```python
from build123d import *

# Parameters (mm, degrees)
EXTRUIR_L_MINA1_DEPTH           = 25
REDONDEO1_R                     = 5
CROQUIS2_R                      = 3
CORTAR_EXTRUIR1_DEPTH           = 41.555257948
REDONDEO2_RADIUS                = 3
REDONDEO2_LENGTH                = 50
REDONDEO3_R                     = 2
REDONDEO1_OF_SIMETR_A1_R        = 5
REDONDEO2_OF_SIMETR_A1_2_RADIUS = 3
REDONDEO2_OF_SIMETR_A1_2_LENGTH = 50
REDONDEO3_OF_SIMETR_A1_R        = 2
TALADRO2_D                      = 5.6
REDONDEO4_R                     = 1


with BuildPart() as part:
    # Croquis1 → Extruir-Lámina1 (new, symmetric)
    with BuildSketch(Plane.XY):
        Polygon((0, 0), (8.029231721, 0), (20, -6.300526927), (31.305467696, -0.350165014), (28.510946527, 4.959321914), (20, 0.479789229), (9.511803576, 6), (0, 6), align=None)
    extruir_l_mina1 = extrude(amount=EXTRUIR_L_MINA1_DEPTH, both=True)

    # Redondeo1
    redondeo1_edges = [part.edges().sort_by_distance(p)[0] for p in [
        (20, 0.479789229, 0),
    ]]
    fillet(redondeo1_edges, radius=REDONDEO1_R)

    # Croquis2 → Cortar-Extruir1 (cut, symmetric)
    with BuildSketch(Plane.XY):
        with Locations((20, -6.300526927)):
            Circle(CROQUIS2_R)
    cortar_extruir1 = extrude(amount=CORTAR_EXTRUIR1_DEPTH, both=True, mode=Mode.SUBTRACT)

    # Redondeo2: full round fillet: the end face becomes a half cylinder, R = half its width
    redondeo2_face = Plane((29.908207112, 2.30457845, 0), x_dir=(0, 0, 1), z_dir=(0.884914487987, 0.465753528113, 0))  # on the end face: x along it, z out of the body
    redondeo2_slab = redondeo2_face.offset(-REDONDEO2_RADIUS / 2) * Box(REDONDEO2_LENGTH, 2 * REDONDEO2_RADIUS, REDONDEO2_RADIUS, mode=Mode.PRIVATE)  # the body's end, R deep
    redondeo2_round = Plane((27.253463648, 0.907317866, 0), x_dir=(0.884914487987, 0.465753528113, 0), z_dir=(0, 0, 1)) * Cylinder(REDONDEO2_RADIUS, REDONDEO2_LENGTH, mode=Mode.PRIVATE)  # its axis R under the face
    add(redondeo2_slab - redondeo2_round, mode=Mode.SUBTRACT)

    # Redondeo3
    redondeo3_edges = [part.edges().sort_by_distance(p)[0] for p in [
        (22.654743464, -4.903266343, 0),
        (17.345256536, -4.903266343, 0),
    ]]
    fillet(redondeo3_edges, radius=REDONDEO3_R)

    # Simetría1: Extruir-Lámina1, Cortar-Extruir1 across plane
    add(extruir_l_mina1.mirror(Plane(origin=(0, 0, 0), x_dir=(0, 0, 1), z_dir=(1, 0, 0))))
    add(cortar_extruir1.mirror(Plane(origin=(0, 0, 0), x_dir=(0, 0, 1), z_dir=(1, 0, 0))), mode=Mode.SUBTRACT)

    # Redondeo1 of Simetría1
    redondeo1_of_simetr_a1_edges = [part.edges().sort_by_distance(p)[0] for p in [
        (-20, 0.479789229, 0),
    ]]
    fillet(redondeo1_of_simetr_a1_edges, radius=REDONDEO1_OF_SIMETR_A1_R)

    # Redondeo2 of Simetr_a1 2: full round fillet: the end face becomes a half cylinder, R = half its width
    redondeo2_of_simetr_a1_2_face = Plane((-29.908207112, 2.30457845, 0), x_dir=(0, 0, 1), z_dir=(-0.884914487987, 0.465753528113, 0))  # on the end face: x along it, z out of the body
    redondeo2_of_simetr_a1_2_slab = redondeo2_of_simetr_a1_2_face.offset(-REDONDEO2_OF_SIMETR_A1_2_RADIUS / 2) * Box(REDONDEO2_OF_SIMETR_A1_2_LENGTH, 2 * REDONDEO2_OF_SIMETR_A1_2_RADIUS, REDONDEO2_OF_SIMETR_A1_2_RADIUS, mode=Mode.PRIVATE)  # the body's end, R deep
    redondeo2_of_simetr_a1_2_round = Plane((-27.253463648, 0.907317866, 0), x_dir=(-0.884914487987, 0.465753528113, 0), z_dir=(0, 0, 1)) * Cylinder(REDONDEO2_OF_SIMETR_A1_2_RADIUS, REDONDEO2_OF_SIMETR_A1_2_LENGTH, mode=Mode.PRIVATE)  # its axis R under the face
    add(redondeo2_of_simetr_a1_2_slab - redondeo2_of_simetr_a1_2_round, mode=Mode.SUBTRACT)

    # Redondeo3 of Simetría1
    redondeo3_of_simetr_a1_edges = [part.edges().sort_by_distance(p)[0] for p in [
        (-22.654743464, -4.903266343, 0),
        (-17.345256536, -4.903266343, 0),
    ]]
    fillet(redondeo3_of_simetr_a1_edges, radius=REDONDEO3_OF_SIMETR_A1_R)

    # Taladro2 (through all)
    with Locations(Plane(origin=(0, 6, 0), x_dir=(1, 0, 0), z_dir=(0, 1, 0))):
        with Locations((0, 15), (0, -15)):
            Hole(TALADRO2_D / 2)

    # Croquis5 → Revolución1 (revolve)
    with BuildSketch(Plane.XY, mode=Mode.PRIVATE) as revoluci_n1_sk:
        Polygon((0, 0), (0, 20), (10, 20), (10, 16), (4, 16), (4, 0), align=None)
    revolve(revoluci_n1_sk.sketch.rotate(Axis((0, 0, 0), (0, 1, 0)), 90), axis=Axis((0, 0, 0), (0, 1, 0)))

    # Redondeo4
    redondeo4_edges = [part.edges().sort_by_distance(p)[0] for p in [
        (0, 20, 10),
        (0, 16, 10),
        (0, 16, 4),
    ]]
    fillet(redondeo4_edges, radius=REDONDEO4_R)


solid = part.part
```
Work out the finished part from the listing and answer in its coordinate system (mm). A direction names the side the tool comes from. Give positions to 0.01 mm unless a question says otherwise; leave off trailing zeros. Order: outer loops, then holes, each group sorted by start corner. A loop starts at its lowest first (then second) coordinate and runs counter-clockwise, first axis right, second up. Notation, with made-up numbers: (-29, -37.75) -> (27, -37.75) arc R22 ccw to (27, -18.75) -> close; hole circle Ø11 at (-12, 51). An arc over 180 degrees is marked (long way). Answer as CSV lines item,"result". Start each with the question number.
(1) Section A-A, the plane z = -15 is taken. Write down the section's boundary in (x, y), plus the area to 3 significant figures.
(2) For a pull along X with two mould halves and no side action, classify faces 1 (the flat face through (0, 1, 25)), 2 (the cylindrical face through (-17.082, -4.386, 0.35)), 3 (the cylindrical face through (3.905, 10.437, 0.867)) as released by +X, released by -X, zero draft, split by the parting line, or undercut.
(3) Section B-B, the plane x = 0 is taken. Write down the section's boundary in (y, z), plus the area to 3 significant figures.
(4) Each of these flat-tipped pins is pushed along its axis until it touches: pin 1 Ø8 at (x, z) = (-1.5, 4.5) entering from -Y; pin 2 Ø9 at (x, z) = (0, 15) entering from +Y; pin 3 Ø1.5 at (y, z) = (2, -15) entering from +X. Where does it stop, or does it pass through?
(5) Section D-D, the plane y = 14 is taken. Write down the section's boundary in (x, z), plus the area to 3 significant figures.
(6) Which of the six approach directions +Z, -Z, +X, -X, +Y, -Y give full straight-line access (tool end or side, diameter ignored) to faces 4 (the flat face through (4, 16, -4)), 5 (the flat face through (24.12, 2.65, 0.35)), 6 (the cylindrical face through (0, 18, 10)), 7 (the flat face through (11.932, -2.054, 0.35))?
(7) Consider line 1 along Z through (x, y) = (0, 4.65); line 2 along X through (y, z) = (1.8, 15); line 3 along Y through (x, z) = (-4, -6). Determine where each line is inside the solid, lowest interval first.
Entries:
1,outline,"(-28.65, -1.75) -> (-24.06, -4.17) arc R2 ccw to (-21.87, -3.96) arc R3 cw to (-18.13, -3.96) arc R2 ccw to (-15.94, -4.17) -> (-8.03, 0) -> (-2.8, 0) -> (-2.8, 6) -> (-9.51, 6) -> (-17.67, 1.71) arc R5 cw to (-22.33, 1.71) -> (-25.86, 3.56) arc R3 ccw to start; (2.8, 0) -> (8.03, 0) -> (15.94, -4.17) arc R2 ccw to (18.13, -3.96) arc R3 cw to (21.87, -3.96) arc R2 ccw to (24.06, -4.17) -> (28.65, -1.75) arc R3 ccw to (25.86, 3.56) -> (22.33, 1.71) arc R5 cw to (17.67, 1.71) -> (9.51, 6) -> (2.8, 6) -> close"
1,area,"331 mm²"
2,face 1,"zero draft"
2,face 2,"undercut"
2,face 3,"split by the parting line"
3,outline,"(0, -25) -> (6, -25) -> (6, -17.8) -> (0, -17.8) -> close; (0, -12.2) -> (6, -12.2) -> (6, -4) -> (15, -4) arc R1 cw to (16, -5) -> (16, -9) arc R1 ccw to (17, -10) -> (19, -10) arc R1 ccw to (20, -9) -> (20, 9) arc R1 ccw to (19, 10) -> (17, 10) arc R1 ccw to (16, 9) -> (16, 5) arc R1 cw to (15, 4) -> (6, 4) -> (6, 12.2) -> (0, 12.2) -> close; (0, 17.8) -> (6, 17.8) -> (6, 25) -> (0, 25) -> close"
3,area,"392 mm²"
4,pin 1,"y = 0"
4,pin 2,"y = 6"
4,pin 3,"x = 30.23"
5,outline,"circle Ø8 at (0, 0)"
5,area,"50.3 mm²"
6,face 4,"none"
6,face 5,"+Z, -Z, +Y"
6,face 6,"+Y"
6,face 7,"+Z, -Z, -Y"
7,line 1,"-25 to -17.8, -12.2 to 12.2, 17.8 to 25"
7,line 2,"-30.12 to -22.51, -17.49 to -2.8, 2.8 to 17.49, 22.51 to 30.12"
7,line 3,"0 to 6, 16 to 20"
